For this review, take the finished solid that the model builds, in its own axes (mm). Face numbers are marked on the shaded views. A direction names the side the tool comes from. Give positions to 0.01 mm unless a question says otherwise; leave off trailing zeros. Order: outer loops, then holes, each group sorted by start corner. A loop starts at its lowest first (then second) coordinate and runs counter-clockwise, first axis right, second up. Notation, with made-up numbers: (72, 64.5) -> (77, 64.5) arc R35 cw to (77, 100.5) -> close; hole circle Ø10 at (-20, 42). An arc over 180 degrees is marked (long way). Use CSV: the item, a comma, the result in double quotes. Start each with the question number.
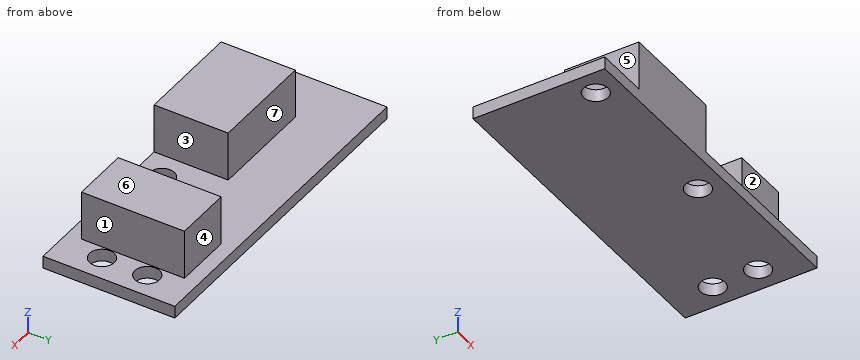
```python
from build123d import *

# Parameters (mm, degrees)
SKETCH027_W     = 40.5
SKETCH027_H     = 16
PAD017_DEPTH    = 1.5
SKETCH028_R     = 1.5
POCKET009_DEPTH = 1.501
SKETCH029_W     = 12.8
SKETCH029_H     = 9
SKETCH029_W_2   = 7
SKETCH029_H_2   = 12.5
PAD018_DEPTH    = 6


with BuildPart() as part:
    # Sketch027 → Pad017 (new body)
    with BuildSketch(Plane.XY):
        with Locations((20.25, 8)):
            Rectangle(SKETCH027_W, SKETCH027_H)
    extrude(amount=PAD017_DEPTH)

    # Sketch028 (on Face6 of Pad017) → Pocket009 (cut, through all)
    with BuildSketch(Plane.XY.offset(1.5)):
        with Locations((3, 3)):
            Circle(SKETCH028_R)
        with Locations((22.5, 3)):
            Circle(SKETCH028_R)
        with Locations((37.5, 10.75)):
            Circle(SKETCH028_R)
        with Locations((37.5, 5.25)):
            Circle(SKETCH028_R)
    extrude(amount=-POCKET009_DEPTH, mode=Mode.SUBTRACT)

    # Sketch029 (on Face5 of Pocket009) → Pad018 (join)
    with BuildSketch(Plane.XY.offset(1.5)):
        with Locations((12.9, 4.5)):
            Rectangle(SKETCH029_W, SKETCH029_H)
        with Locations((32.4, 8)):
            Rectangle(SKETCH029_W_2, SKETCH029_H_2)
    extrude(amount=PAD018_DEPTH)


solid = part.part
```
1. To check wall thickness, follow L1, parallel to Y at x = 37.5, z = 1.15; L2, parallel to X at y = 4.75, z = 5; L3, parallel to Y at x = 13, z = 7. State the ranges of each line that lie inside material, in increasing order. Write a range as [from, to].
2. Consider section B-B (z = 6.5). State the section outline as (x, y) points, plus the area to 3 significant figures.
3. Consider section A-A (x = 22.5). State the section outline as (y, z) points, plus the area to 3 significant figures.
4. Consider section D-D (x = 37.5). State the section outline as (y, z) points, plus the area to 3 significant figures.
5. Consider section C-C (y = 5.25). State the section outline as (x, z) points, plus the area to 3 significant figures.
6. Draft analysis for pull direction X (two halves, no side actions). For the marked faces 1, 2 and 3, state which applies: +X half, -X half, draft (parallel to the pull), parting line (faces both ways), or undercut.
7. Clearance check with flat-ended pins moving along their axes: P1, Ø3, axis at y = 4, z = 5, coming from the -X side; P2, Ø1, axis at x = 31.5, z = 2.5, coming from the +Y side; P3, Ø1.5, axis at x = 16, y = 9, coming from the -Z side; P4, Ø5, axis at x = 23.5, y = 5.5, coming from the +Z side. State where each tip first meets the part, or that it passes through.
8. For the marked faces 4, 5, 6 and 7, list the 3-axis set-ups (+Z, -Z, +X, -X, +Y, -Y) from which the entire face can be reached by the end or side of a thin tool; tool diameter is ignored.
Answer list:
1,L1,"[0, 3.75], [6.75, 9.25], [12.25, 16]"
1,L2,"[6.5, 19.3], [28.9, 35.9]"
1,L3,"[0, 9]"
2,outline,"(6.5, 0) -> (19.3, 0) -> (19.3, 9) -> (6.5, 9) -> close; (28.9, 1.75) -> (35.9, 1.75) -> (35.9, 14.25) -> (28.9, 14.25) -> close"
2,area,"203 mm2"
3,outline,"(0, 0) -> (1.5, 0) -> (1.5, 1.5) -> (0, 1.5) -> close; (4.5, 0) -> (16, 0) -> (16, 1.5) -> (4.5, 1.5) -> close"
3,area,"19.5 mm2"
4,outline,"(0, 0) -> (3.75, 0) -> (3.75, 1.5) -> (0, 1.5) -> close; (6.75, 0) -> (9.25, 0) -> (9.25, 1.5) -> (6.75, 1.5) -> close; (12.25, 0) -> (16, 0) -> (16, 1.5) -> (12.25, 1.5) -> close"
4,area,"15.0 mm2"
5,outline,"(0, 0) -> (36, 0) -> (36, 1.5) -> (35.9, 1.5) -> (35.9, 7.5) -> (28.9, 7.5) -> (28.9, 1.5) -> (19.3, 1.5) -> (19.3, 7.5) -> (6.5, 7.5) -> (6.5, 1.5) -> (0, 1.5) -> close; (39, 0) -> (40.5, 0) -> (40.5, 1.5) -> (39, 1.5) -> close"
5,area,"175 mm2"
6,face 1,"+X half"
6,face 2,"draft"
6,face 3,"undercut"
7,P1,"x = 6.5"
7,P2,"y = 14.25"
7,P3,"z = 0"
7,P4,"z = 1.5"
8,face 4,"+Z, +X, -X, +Y"
8,face 5,"+Z, -X, +Y, -Y"
8,face 6,"+Z, +X, -X, +Y, -Y"
8,face 7,"+Z, -X, +Y"
